Verification items for the finished model (mm, model axes). Face numbers are marked on the shaded views. A direction names the side the tool comes from. Coordinates: 2 decimals unless noted, no trailing zeros. Order: outer loops, then holes, each group sorted by start corner. A loop starts at its lowest first (then second) coordinate and runs counter-clockwise, first axis right, second up. Notation, with made-up numbers: M 29.5,34.5 L 67.5,34.5 A13 ccw 67.5,38.5 Z; hole C 53.5,-32.75 d4. An arc over 180 degrees is marked long. Return JSON: item names as keys, results as strings. Group by question number.
1. Section check C-C, the plane x = -31.5. Record the cut outline in (y, z), plus the area to 3 significant figures.
2. Section check D-D, the plane z = 25. Record the cut outline in (x, y).
3. Gauge pin test, flat ends, axial feed: pin 1 (20 mm diameter, centred on x = 172, y = 24.5, fed in from +Z); pin 2 (12 mm diameter, centred on x = 173, y = 28.5, fed in from -Z); pin 3 (3 mm diameter, centred on x = 18, z = 34.5, fed in from +Y). Record the tip position at first contact, or that the pin passes through.
4. Material ranges on line 1 along Y through (x, z) = (189, 0); line 2 along X through (y, z) = (17.5, 1); line 3 along Y through (x, z) = (92, 28), recorded low to high.
5. Set-up check for the marked faces 1, 2, 3, 4 and 5: record each of +Z, -Z, +X, -X, +Y, -Y from which the full face is reachable in a straight line by a thin tool's end or side.
6. Mould release check, pull along Y, two halves, no side actions. Record for the marked faces 6, 7, 8 and 9: +Y half, -Y half, draft (parallel to the pull), parting line (faces both ways), or undercut.
7. Section check A-A, the plane y = 17.5. Record the cut outline in (x, z), plus the area to 3 significant figures.
8. Section check B-B, the plane z = 9. Record the cut outline in (x, y), plus the area to 3 significant figures.
```python
from build123d import *

# Parameters (mm, degrees)
SKETCH1_W           = 400
SKETCH1_H           = 100
BOSS_EXTRUDE1_DEPTH = 5
SKETCH6_R           = 15.180517927
BOSS_EXTRUDE2_DEPTH = 40
SKETCH7_R           = 0.320199733
BOSS_EXTRUDE3_DEPTH = 0.5


with BuildPart() as part:
    # Sketch1 → Boss-Extrude1 (new body)
    with BuildSketch(Plane(origin=(0, 0, 0), x_dir=(1, 0, 0), z_dir=(0, 1, 0))):
        Rectangle(SKETCH1_W, SKETCH1_H)
    extrude(amount=BOSS_EXTRUDE1_DEPTH)

    # Sketch6 → Boss-Extrude2 (add)
    with BuildSketch(Plane(origin=(200, 0, 0), x_dir=(0, 0, -1), z_dir=(1, 0, 0))):
        with BuildLine():
            Line((-20, 45), (-20, 5))
            Line((-20, 5), (20, 5))
            Line((20, 5), (20, 45))
            ThreePointArc((20, 45), (0, 65), (-20, 45))
        make_face()
        with Locations((0, 45)):
            Circle(SKETCH6_R, mode=Mode.SUBTRACT)
    boss_extrude2 = extrude(amount=-BOSS_EXTRUDE2_DEPTH)

    # Mirror1: Boss-Extrude2 across plane
    add(boss_extrude2.mirror(Plane(origin=(0, 0, 0), x_dir=(0, 0, 1), z_dir=(1, 0, 0))))

    # Sketch7 → Boss-Extrude3 (add)
    with BuildSketch(Plane(origin=(0, 5, 0), x_dir=(1, 0, 0), z_dir=(0, 1, 0))):
        Circle(SKETCH7_R)
    extrude(amount=BOSS_EXTRUDE3_DEPTH)


solid = part.part
```
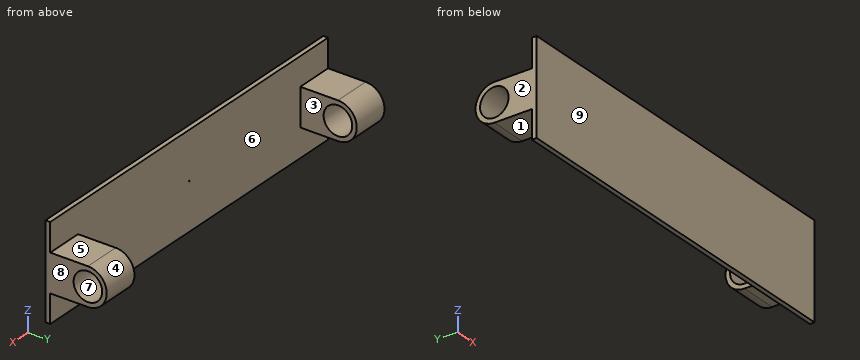
Answers follow:
{
 "1": {"outline": "M 0,-50 L 5,-50 L 5,50 L 0,50 Z", "area": "500 mm^2"},
 "2": {"outline": "M -200,0 L 200,0 L 200,5 L -200,5 Z"},
 "3": {"pin 1": "z = 20", "pin 2": "z = -20", "pin 3": "y = 5"},
 "4": {"line 1": "0 to 29.82, 60.18 to 65", "line 2": "-200 to -160, 160 to 200", "line 3": "0 to 5"},
 "5": {"face 1": "-Z, +X, -X, +Y", "face 2": "+Z, -Z, -X, +Y, -Y", "face 3": "+Z, -Z, +Y", "face 4": "+X, -X, +Y", "face 5": "+Z, +X, -X, +Y"},
 "6": {"face 6": "+Y half", "face 7": "undercut", "face 8": "draft", "face 9": "-Y half"},
 "7": {"outline": "M -200,-20 L -160,-20 L -160,20 L -200,20 Z; M 160,-20 L 200,-20 L 200,20 L 160,20 Z", "area": "3,200 mm^2"},
 "8": {"outline": "M -200,0 L 200,0 L 200,32.78 L 160,32.78 L 160,5 L -160,5 L -160,32.78 L -200,32.78 Z; M -200,57.22 L -160,57.22 L -160,62.86 L -200,62.86 Z; M 160,57.22 L 200,57.22 L 200,62.86 L 160,62.86 Z", "area": "4,670 mm^2"}
}
